Work out the finished part from the listing and answer in its coordinate system (mm). A direction names the side the tool comes from. Coordinates: 2 decimals unless noted, no trailing zeros. Loops run counter-clockwise (first coordinate to the right, second up) from the corner with the lowest first, then second, coordinate; pieces in that order, holes last. Notation, with made-up numbers: (21.5, 82.25) -> (45.5, 82.25) arc R20 cw to (45.5, 86.25) -> close; hole circle Ø3 at (0, 3.5). An arc over 180 degrees is marked (long way). One line per question, with ' | ' between items.
```python
from build123d import *

# Parameters (mm, degrees)
F0_R     = 6.35
F0_R_2   = 3.175
F0_R_3   = 26.9875
F1_DEPTH = 3.175


# Not quite as in the source:
# - a feature names something its author has since deleted; it is built from what else it names


with BuildPart() as f1:
    # F0 (on Front) → F1 (new body)
    with BuildSketch(Plane.XZ):
        with BuildLine():
            ThreePointArc((-43.4258934254, 9.4865315159), (-40.2925849359, 18.769925391), (-35.2015661866, 27.1413381765))
            Line((-35.2015661866, 27.1413381765), (-95.2689163392, 37.7723748329))
            ThreePointArc((-95.2689163392, 37.7723748329), (-98.7721627257, 39.6581308221), (-100.4657668126, 43.2582025009))
            ThreePointArc((-100.4657668126, 43.2582025009), (-121.3252913638, 62.0407471137), (-139.3392654958, 40.5140083313))
            Line((-139.3392654958, 40.5140083313), (-138.3529874387, 31.3088718833))
            ThreePointArc((-138.3529874387, 31.3088718833), (-134.5315509232, 21.8873221018), (-126.2516022963, 15.9872010809))
            Line((-126.2516022963, 15.9872010809), (-42.4180155898, -13.285874206))
            ThreePointArc((-42.4180155899, -13.285874206), (-44.3727417421, -2.6195973531), (-43.6866122567, 8.2025855396))
            ThreePointArc((-43.6866122567, 8.2025855396), (-48.388636459, 2.3785824935), (-55.8537619567, 1.8309107075))
            Line((-55.8537619567, 1.8309107075), (-110.4577448757, 20.8975708106))
            ThreePointArc((-110.4577448757, 20.8975708106), (-111.1735466188, 21.086419267), (-111.8513183434, 21.3841798493))
            ThreePointArc((-111.8513183434, 21.3841798493), (-114.2200668687, 26.7082159188), (-109.6486913125, 30.321919721))
            ThreePointArc((-109.6486913125, 30.321919721), (-108.7795274506, 30.2493985469), (-107.9382701007, 30.0192003476))
            Line((-107.9382701007, 30.0192003476), (-51.5976439548, 20.0477389749))
            ThreePointArc((-51.5976439548, 20.0477389749), (-51.1132512592, 19.9749597914), (-50.6333036668, 19.8770649411))
            ThreePointArc((-50.6333036668, 19.8770649411), (-45.0232212062, 16.073525101), (-43.4258934254, 9.4865315159))
        make_face()
        with Locations((-120.6001266837, 50.3768287599)):
            Circle(F0_R, mode=Mode.SUBTRACT)
        with BuildLine():
            ThreePointArc((35.2015661866, 27.1413381765), (0, 44.45), (-35.2015661866, 27.1413381765))
            ThreePointArc((-35.2015661866, 27.1413381765), (-40.2925849359, 18.769925391), (-43.4258934254, 9.4865315159))
            ThreePointArc((-43.4258934254, 9.4865315159), (-43.533872992, 8.8400140623), (-43.6866122567, 8.2025855396))
            ThreePointArc((-43.6866122567, 8.2025855396), (-44.3727417421, -2.6195973531), (-42.4180155899, -13.285874206))
            ThreePointArc((-42.4180155899, -13.285874206), (0, -44.45), (42.4180155899, -13.285874206))
            ThreePointArc((42.4180155899, -13.285874206), (43.9390674285, -6.7201825508), (44.45, 0))
            ThreePointArc((44.45, 0), (44.2587415931, 4.1190159741), (43.6866122567, 8.2025855396))
            ThreePointArc((43.6866122567, 8.2025855396), (43.533872992, 8.8400140623), (43.4258934254, 9.4865315159))
            ThreePointArc((43.4258934254, 9.4865315159), (40.2925849359, 18.769925391), (35.2015661866, 27.1413381765))
        make_face()
        with Locations((0, -34.925)):
            Circle(F0_R_2, mode=Mode.SUBTRACT)
        with Locations((-30.2459372272, -17.4625)):
            Circle(F0_R_2, mode=Mode.SUBTRACT)
        Circle(F0_R_3, mode=Mode.SUBTRACT)
        with Locations((30.2459372272, -17.4625)):
            Circle(F0_R_2, mode=Mode.SUBTRACT)
        with Locations((-30.2459372272, 17.4625)):
            Circle(F0_R_2, mode=Mode.SUBTRACT)
        with Locations((0, 34.925)):
            Circle(F0_R_2, mode=Mode.SUBTRACT)
        with Locations((30.2459372272, 17.4625)):
            Circle(F0_R_2, mode=Mode.SUBTRACT)
        with BuildLine():
            Line((95.2689163392, 37.7723748329), (35.2015661866, 27.1413381765))
            ThreePointArc((35.2015661866, 27.1413381765), (40.2925849359, 18.769925391), (43.4258934254, 9.4865315159))
            ThreePointArc((43.4258934254, 9.4865315159), (45.0232212062, 16.073525101), (50.6333036668, 19.8770649411))
            ThreePointArc((50.6333036668, 19.8770649411), (51.1132512592, 19.9749597914), (51.5976439548, 20.0477389749))
            Line((51.5976439548, 20.0477389749), (107.9382701008, 30.0192003476))
            ThreePointArc((107.9382701008, 30.0192003476), (108.7795274506, 30.2493985469), (109.6486913125, 30.321919721))
            ThreePointArc((109.6486913125, 30.321919721), (114.2200668687, 26.7082159188), (111.8513183434, 21.3841798493))
            ThreePointArc((111.8513183434, 21.3841798493), (111.1735466188, 21.086419267), (110.4577448757, 20.8975708106))
            Line((110.4577448757, 20.8975708106), (55.8537619567, 1.8309107075))
            ThreePointArc((55.8537619567, 1.8309107075), (48.388636459, 2.3785824935), (43.6866122567, 8.2025855396))
            ThreePointArc((43.6866122567, 8.2025855396), (44.2587415931, 4.1190159741), (44.45, 0))
            ThreePointArc((44.45, 0), (43.9390674285, -6.7201825508), (42.4180155899, -13.285874206))
            Line((42.4180155898, -13.285874206), (126.2516022963, 15.9872010809))
            ThreePointArc((126.2516022963, 15.9872010809), (134.5315509232, 21.8873221018), (138.3529874387, 31.3088718833))
            Line((138.3529874387, 31.3088718833), (139.3392654958, 40.5140083313))
            ThreePointArc((139.3392654958, 40.5140083313), (121.3252913638, 62.0407471137), (100.4657668126, 43.2582025009))
            ThreePointArc((100.4657668126, 43.2582025009), (98.7721627257, 39.6581308221), (95.2689163392, 37.7723748329))
        make_face()
        with Locations((120.6001266837, 50.3768287599)):
            Circle(F0_R, mode=Mode.SUBTRACT)
    extrude(amount=F1_DEPTH)


solid = f1.part
```
1) The mould has two halves that part along Z. Classify faces 1 (the face through (134.44, -1.57, 21.77)), 2 (the face through (-11, 0, 33)), 3 (the face through (-82.77, -1.57, 11.23)), 4 (the face through (33.274, -1.565, 18.416)): released by +Z, released by -Z, zero draft, split by the parting line, or undercut.
Check values:
face 1: released by -Z | face 2: zero draft | face 3: undercut | face 4: undercut
2) Find section A-A (x = 0). State how many separate pieces and enclosed holes the cut face has, plus the area to 3 significant figures.
Check values:
separate pieces: 4 | enclosed holes: 0 | area: 70.6 mm^2
3) Flat-ended cylindrical pins translate along their axes: pin 1 (12 mm diameter, centred on x = -42, z = 16.5, fed in from +Y); pin 2 (3 mm diameter, centred on x = -97, z = 19, fed in from +Y). Find the tip coordinate at first contact, or state that the pin passes through.
Check values:
pin 1: stops at y = 0 | pin 2: passes through
4) Find section B-B (x = -92). Write down the section's boundary in (y, z) (3 decimals), plus the area to 3 significant figures.
Check values:
outline: (-3.175, 4.027) -> (0, 4.027) -> (0, 14.452) -> (-3.175, 14.452) -> close; (-3.175, 27.198) -> (0, 27.198) -> (0, 37.194) -> (-3.175, 37.194) -> close | area: 64.8 mm^2
5) Find the intervals of material crossed by line 1 along Z through (x, y) = (0, -1.4); line 2 along X through (y, z) = (-0.6, 44.5); line 3 along X through (y, z) = (-0.8, 52.5), in increasing order.
Check values:
line 1: z = -44.45 to -38.1, -31.75 to -26.99, 26.99 to 31.75, 38.1 to 44.45 | line 2: x = -139.36 to -123.01, -118.19 to -100.55, 100.55 to 118.19, 123.01 to 139.36 | line 3: x = -136.74 to -126.58, -114.62 to -103.16, 103.16 to 114.62, 126.58 to 136.74
6) For faces 5 (the face through (-11, -3.175, 33)), 6 (the face through (-80.162, -1.565, 25.103)), 7 (the face through (98.81, -1.57, 39.7)), determine the directions among +Z, -Z, +X, -X, +Y, -Y from which every point of the face is accessible in a straight line to the end or side of a thin tool.
Check values:
face 5: +Z, -Z, +X, -X, -Y | face 6: +Y, -Y | face 7: +Z, +Y, -Y
